Check sheet for the drawn part. Datum: minimum x, y, z corner. Units: mm. A direction names the side the tool comes from. Round coordinates to 2 decimals unless told otherwise and drop trailing zeros. Write each loop counter-clockwise with the first axis right and the second up, starting at its lowest first coordinate (ties: lowest second). Pieces come first, ordered by that corner, then holes. Notation, with made-up numbers: M -4.75,-27.5 L 47.25,-27.5 A10 cw 47.25,-21.5 Z; hole C -34.75,31.5 d5. An arc over 180 degrees is marked long. Use a Markdown table: item, result.
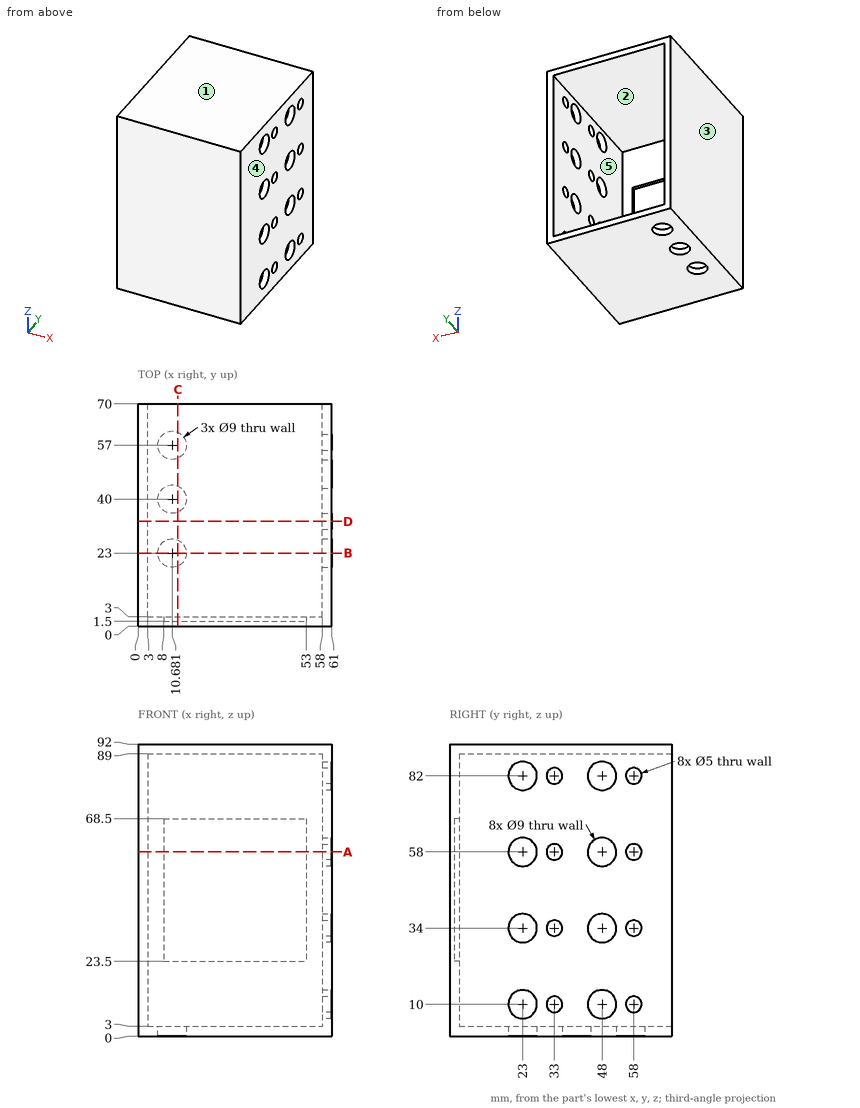
Item 1: Go/stop test with flat-tipped pins: pin 1 (3 mm diameter, centred on y = 33, z = 58, fed in from +X); pin 2 (1 mm diameter, centred on x = 33.5, z = 61.5, fed in from +Y). Record where each tip stops, or that it passes through.
Outcome:
| item | result |
|---|---|
| pin 1 | stops at x = 3 |
| pin 2 | stops at y = 1.5 |
Item 2: Cross-section at B-B, the plane y = 23. Record the cut outline in (x, z).
Outcome:
| item | result |
|---|---|
| outline | M 0,0 L 6.18,0 L 6.18,3 L 3,3 L 3,89 L 58,89 L 58,86.5 L 61,86.5 L 61,92 L 0,92 Z; M 15.18,0 L 61,0 L 61,5.5 L 58,5.5 L 58,3 L 15.18,3 Z; M 58,14.5 L 61,14.5 L 61,29.5 L 58,29.5 Z; M 58,38.5 L 61,38.5 L 61,53.5 L 58,53.5 Z; M 58,62.5 L 61,62.5 L 61,77.5 L 58,77.5 Z |
Item 3: Cross-section at D-D, the plane y = 33. Record the cut outline in (x, z).
Outcome:
| item | result |
|---|---|
| outline | M 0,0 L 61,0 L 61,7.5 L 58,7.5 L 58,3 L 3,3 L 3,89 L 58,89 L 58,84.5 L 61,84.5 L 61,92 L 0,92 Z; M 58,12.5 L 61,12.5 L 61,31.5 L 58,31.5 Z; M 58,36.5 L 61,36.5 L 61,55.5 L 58,55.5 Z; M 58,60.5 L 61,60.5 L 61,79.5 L 58,79.5 Z |
Item 4: Mould release check, pull along X, two halves, no side actions. Record for the marked faces 3, 4 and 5: +X half, -X half, draft (parallel to the pull), parting line (faces both ways), or undercut.
Outcome:
| item | result |
|---|---|
| face 3 | -X half |
| face 4 | +X half |
| face 5 | undercut |
Item 5: Cross-section at A-A, the plane z = 58. Record the cut outline in (x, y).
Outcome:
| item | result |
|---|---|
| outline | M 0,0 L 61,0 L 61,18.5 L 58,18.5 L 58,3 L 53,3 L 53,1.5 L 8,1.5 L 8,3 L 3,3 L 3,70 L 0,70 Z; M 58,27.5 L 61,27.5 L 61,30.5 L 58,30.5 Z; M 58,35.5 L 61,35.5 L 61,43.5 L 58,43.5 Z; M 58,52.5 L 61,52.5 L 61,55.5 L 58,55.5 Z; M 58,60.5 L 61,60.5 L 61,70 L 58,70 Z |
Item 6: Cross-section at C-C, the plane x = 12.5. Record the cut outline in (y, z).
Outcome:
| item | result |
|---|---|
| outline | M 0,0 L 18.88,0 L 18.88,3 L 3,3 L 3,23.5 L 1.5,23.5 L 1.5,68.5 L 3,68.5 L 3,89 L 70,89 L 70,92 L 0,92 Z; M 27.12,0 L 35.88,0 L 35.88,3 L 27.12,3 Z; M 44.12,0 L 52.88,0 L 52.88,3 L 44.12,3 Z; M 61.12,0 L 70,0 L 70,3 L 61.12,3 Z |
Item 7: Material ranges on line 1 along Y through (x, z) = (59.05, 10); line 2 along X through (y, z) = (5, 21); line 3 along Z through (x, y) = (16, 33.5), recorded low to high. Write a range as from..to.
Outcome:
| item | result |
|---|---|
| line 1 | y = 0..18.5, 27.5..30.5, 35.5..43.5, 52.5..55.5, 60.5..70 |
| line 2 | x = 0..3, 58..61 |
| line 3 | z = 0..3, 89..92 |
Item 8: Access from +Z, -Z, +X, -X, +Y, -Y to the whole of each face (thin tool, end or side, straight path). Record for the marked faces 1 and 2.
Outcome:
| item | result |
|---|---|
| face 1 | +Z, +X, -X, +Y, -Y |
| face 2 | +Y |
